For this review, take the finished solid that the model builds, in its own axes (mm). A direction names the side the tool comes from. Give positions to 0.01 mm unless a question says otherwise; leave off trailing zeros. Order: outer loops, then holes, each group sorted by start corner. A loop starts at its lowest first (then second) coordinate and runs counter-clockwise, first axis right, second up. Notation, with made-up numbers: (74.25, 54) - (99.25, 54) arc R11 cw to (99.25, 71) - close; hole circle Ø3 at (-11, -14). An arc over 180 degrees is marked (long way). One line per item, written item: value.
```python
from build123d import *

# Parameters (mm, degrees)
F1_DEPTH = 25


with BuildPart() as f1:
    # F0 (on Top) → F1 (new body)
    with BuildSketch(Plane.XY):
        with BuildLine():
            Line((0, 5), (0, 0))
            Line((0, 0), (29, 0))
            Line((29, 0), (30, 0))
            Line((30, 0), (30, 5))
            Line((30, 5), (50, 5))
            Line((50, 5), (50, 0))
            Line((50, 0), (80, 0))
            Line((80, 0), (80, 5))
            Line((80, 5), (98, 5))
            ThreePointArc((98, 5), (99.414214, 5.585786), (100, 7))
            Line((100, 7), (100, 15))
            Line((100, 15), (76, 35))
            Line((76, 35), (68, 35))
            Line((68, 35), (68, 29))
            Line((68, 29), (60, 29))
            Line((60, 29), (60, 35))
            Line((60, 35), (52, 35))
            Line((52, 35), (52, 29))
            Line((52, 29), (44, 29))
            Line((44, 29), (44, 35))
            Line((44, 35), (36, 35))
            Line((36, 35), (36, 29))
            Line((36, 29), (28, 29))
            Line((28, 29), (28, 35))
            Line((28, 35), (20, 35))
            Line((20, 35), (20, 29))
            Line((20, 29), (12, 29))
            Line((12, 29), (12, 35))
            Line((12, 35), (4, 35))
            Line((4, 35), (-20, 15))
            Line((-20, 15), (-20, 7))
            ThreePointArc((-20, 7), (-19.414214, 5.585786), (-18, 5))
            Line((-18, 5), (0, 5))
        make_face()
        with BuildLine():
            ThreePointArc((29, 15), (27.828427, 12.171573), (25, 11))
            Line((25, 11), (5, 11))
            ThreePointArc((5, 11), (2.171573, 12.171573), (1, 15))
            ThreePointArc((1, 15), (2.171573, 17.828427), (5, 19))
            Line((5, 19), (25, 19))
            ThreePointArc((25, 19), (27.828427, 17.828427), (29, 15))
        make_face(mode=Mode.SUBTRACT)
        with BuildLine():
            ThreePointArc((55, 11), (52.171573, 12.171573), (51, 15))
            ThreePointArc((51, 15), (52.171573, 17.828427), (55, 19))
            Line((55, 19), (75, 19))
            ThreePointArc((75, 19), (77.828427, 17.828427), (79, 15))
            ThreePointArc((79, 15), (77.828427, 12.171573), (75, 11))
            Line((75, 11), (55, 11))
        make_face(mode=Mode.SUBTRACT)
    extrude(amount=F1_DEPTH)


solid = f1.part
```
(1) Draft analysis for pull direction X (two halves, no side actions). For faces 1 (the face through (-19.43, 5.6, 12.32)), 2 (the face through (12, 32, 12)), 3 (the face through (-9, 5, 12)), state which applies: pulls with the +X half, pulls with the -X half, needs draft (parallel to the pull), parting line crosses it, or undercut.
Answers below:
face 1: pulls with the -X half
face 2: undercut
face 3: needs draft
(2) For P1, Ø9, axis at x = -9, z = 6.5, coming from the -Y side; P2, Ø5, axis at y = 31, z = 9, coming from the -X side; P3, Ø1.5, axis at y = 16, z = 5, coming from the -X side, all flat-tipped, find the tip position at first contact; note any pin that passes through.
Answers below:
P1: stops at y = 5
P2: stops at x = -3.8
P3: stops at x = -19.7
(3) Take a section at C-C (x = 34). Write out the cut boundary in (y, z), then the cut area to 3 significant figures.
Answers below:
outline: (5, 0) - (29, 0) - (29, 25) - (5, 25) - close
area: 600 mm^2
(4) Take a section at A-A (x = 53.5). Write out the cut boundary in (y, z), then the cut area to 3 significant figures.
Answers below:
outline: (0, 0) - (11.29, 0) - (11.29, 25) - (0, 25) - close; (18.71, 0) - (35, 0) - (35, 25) - (18.71, 25) - close
area: 690 mm^2
(5) Take a section at B-B (z = 3.25). Give the number of separate pieces and of enclosed holes in the cut face, then the cut area to 3 significant figures.
Answers below:
separate pieces: 1
enclosed holes: 2
area: 2,810 mm^2
(6) Machinability: for faces 4 (the face through (32, 29, 12)), 5 (the face through (89, 5, 12)), 6 (the face through (15, 19, 12)), which of the approach directions +Z, -Z, +X, -X, +Y, -Y give a long, thin tool a straight path to every point of the face, cutting with its end or side? Answer none if there is none.
Answers below:
face 4: +Z, -Z, +Y
face 5: +Z, -Z, +X, -Y
face 6: +Z, -Z
(7) Wall thickness on line 1 (Y direction, x = 55.5, z = 5.5); line 2 (X direction, y = 33.5, z = 17.75); line 3 (X direction, y = 12.5, z = 6.5): over which ranges is each line inside the solid? List them lowest first. Write a range as from..to.
Answers below:
line 1: y = 0..11, 19..35
line 2: x = 2.2..12, 20..28, 36..44, 52..60, 68..77.8
line 3: x = -20..1.88, 28.12..51.88, 78.12..100
(8) Take a section at D-D (y = 24). Write out the cut boundary in (x, z), then the cut area to 3 significant figures.
Answers below:
outline: (-9.2, 0) - (89.2, 0) - (89.2, 25) - (-9.2, 25) - close
area: 2,460 mm^2
